Solid Edge part; units mm, degrees
sketch "Sketch1" plane through (0, 0, 0) normal (0, -1, 0) x (1, 0, 0)
  line L0 (-92.067, 25.1901) -> (-52.067, 25.1901)
  line L1 (-52.067, 25.1901) -> (-52.067, 65.1901)
  line L2 (-52.067, 65.1901) -> (-92.067, 65.1901)
  line L3 (-92.067, 65.1901) -> (-92.067, 25.1901)
  dimension "D1" = 52.067
  dimension "D2" = 52.067
extrude "Protrusion1" add sketch "Sketch1" along normal blind 80
sketch "Sketch2" plane through (-52.067, -75, 45.1901) normal (1, 0, 0) x (0, 1, 0)
  circle A0 centre (-40, 0) radius 5
  line L0 (-5, 20) -> (-50, 7.5)
  line L1 (-50, 7.5) -> (-50, -7.5)
  line L2 (-50, -7.5) -> (-5, -20)
  line L3 (-5, -20) -> (-5, 20)
  dimension "D1" = 50
  dimension "D2" = 40
extrude "ExtrudedProtrusion_2" add sketch "Sketch2" against normal blind 8
mirror "Mirror1" about plane through (-68.067, -90.8694, 45.1901) normal (1, 0, 0) of "ExtrudedProtrusion_2"
hole "Hole_1" at (-92.067, -50, 55.1901) direction (1, 0, 0) diameter 6.35 end up to next
hole "Hole1" at (-92.067, -30, 35.1901) direction (1, 0, 0) diameter 6.35 end up to next
hole "Hole2" at (-92.067, -50, 35.1901) direction (1, 0, 0) diameter 6.35 end up to next
hole "Hole3" at (-92.067, -30, 55.1901) direction (1, 0, 0) diameter 6.35 end up to next
hole "Hole_5" at (-62.067, -30, 65.1901) direction (0, 0, -1) diameter 6.35 end up to next
hole "Hole4" at (-82.067, -30, 65.1901) direction (0, 0, -1) diameter 6.35 end up to next
hole "Hole5" at (-82.067, -70, 65.1901) direction (0, 0, -1) diameter 6.35 end up to next
hole "Hole6" at (-62.067, -70, 65.1901) direction (0, 0, -1) diameter 6.35 end up to next
properties material "Aluminum, 6061-T6"
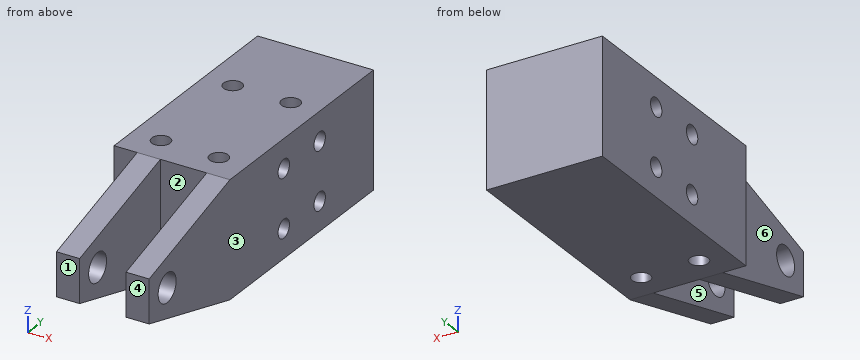
Geometry check sheet. Reference: the model listing, model coordinates, mm. Face numbers are marked on the shaded views. A direction names the side the tool comes from. Round coordinates to 2 decimals unless told otherwise and drop trailing zeros. Write each loop counter-clockwise with the first axis right and the second up, starting at its lowest first coordinate (ties: lowest second). Pieces come first, ordered by that corner, then holes.
Item 1: Section check B-B (x = -89). Record the boundary of the cut face in (y, z) (3 decimals), plus the area to 3 significant figures.
Determined:
outline: (-80, 25.19) - (0, 25.19) - (0, 65.19) - (-80, 65.19) - close; hole circle Ø6.35 at (-50, 35.19); hole circle Ø6.35 at (-50, 55.19); hole circle Ø6.35 at (-30, 35.19); hole circle Ø6.35 at (-30, 55.19)
area: 3,070 mm2
Item 2: Section check A-A (y = -50). Record the boundary of the cut face in (x, z), plus the area to 3 significant figures.
Determined:
outline: (-92.07, 25.19) - (-52.07, 25.19) - (-52.07, 32.02) - (-92.07, 32.02) - close; (-92.07, 38.37) - (-52.07, 38.37) - (-52.07, 52.02) - (-92.07, 52.02) - close; (-92.07, 58.37) - (-52.07, 58.37) - (-52.07, 65.19) - (-92.07, 65.19) - close
area: 1,090 mm2
Item 3: Mould release check, pull along X, two halves, no side actions. Record for the marked faces 1, 2 and 3: +X half, -X half, draft (parallel to the pull), parting line (faces both ways), or undercut.
Determined:
face 1: draft
face 2: undercut
face 3: +X half
Item 4: Go/stop test with flat-tipped pins: pin 1 Ø4 at (y, z) = (-50, 35.19) entering from +X; pin 2 Ø12 at (y, z) = (-94, 54) entering from -X; pin 3 Ø8 at (x, z) = (-66, 55) entering from -Y. Record where each tip stops, or that it passes through.
Determined:
pin 1: passes through
pin 2: stops at x = -84.07
pin 3: stops at y = -80
Item 5: Section check C-C (z = 57). Record the boundary of the cut face in (x, y) (3 decimals), plus the area to 3 significant figures.
Determined:
outline: (-92.067, -80) - (-84.067, -80) - (-84.067, -109.484) - (-76.067, -109.484) - (-76.067, -80) - (-60.067, -80) - (-60.067, -109.484) - (-52.067, -109.484) - (-52.067, -52.609) - (-92.067, -52.609) - close; (-92.067, -47.391) - (-52.067, -47.391) - (-52.067, -32.609) - (-60.257, -32.609) arc R3.175 cw to (-63.877, -32.609) - (-80.257, -32.609) arc R3.175 cw to (-83.877, -32.609) - (-92.067, -32.609) - close; (-92.067, -27.391) - (-83.877, -27.391) arc R3.175 cw to (-80.257, -27.391) - (-63.877, -27.391) arc R3.175 cw to (-60.257, -27.391) - (-52.067, -27.391) - (-52.067, 0) - (-92.067, 0) - close; hole circle Ø6.35 at (-82.067, -70); hole circle Ø6.35 at (-62.067, -70)
area: 3,190 mm2
Item 6: Section check D-D (y = -105). Record the boundary of the cut face in (x, z), plus the area to 3 significant figures.
Determined:
outline: (-84.07, 32.13) - (-76.07, 32.13) - (-76.07, 58.25) - (-84.07, 58.25) - close; (-60.07, 32.13) - (-52.07, 32.13) - (-52.07, 58.25) - (-60.07, 58.25) - close
area: 418 mm2
Item 7: Access from +Z, -Z, +X, -X, +Y, -Y to the whole of each face (thin tool, end or side, straight path). Record for the marked faces 4, 5 and 6.
Determined:
face 4: +Z, -Z, +X, -X, -Y
face 5: +Z, -Z, -Y
face 6: +Z, -Z, -X, -Y
Item 8: Material ranges on line 1 along X through (y, z) = (-70, 39); line 2 along Z through (x, y) = (-73, -51); line 3 along Z through (x, y) = (-61, -30), recorded low to high.
Determined:
line 1: x = -92.07 to -85.24, -78.89 to -65.24, -58.89 to -52.07
line 2: z = 25.19 to 32.18, 38.2 to 52.18, 58.2 to 65.19
line 3: z = 25.19 to 32.02, 38.37 to 52.02
